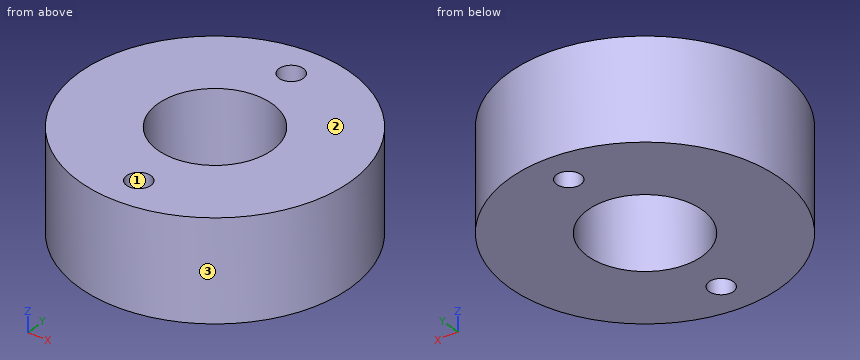
```python
from build123d import *

# Parameters (mm, degrees)
SKETCH1_R                      = 9.45
BOSS_EXTRUDE1_DEPTH            = 7
CUT_EXTRUDE1_REACH             = 17.087
SKETCH2_R                      = 4
TAP_DRILL_FOR_M2_5X0_45_TAP1_D = 1.7


with BuildPart() as part:
    # Sketch1 → Boss-Extrude1 (new body)
    with BuildSketch(Plane.XY):
        Circle(SKETCH1_R)
    extrude(amount=BOSS_EXTRUDE1_DEPTH)

    # Sketch2 → Cut-Extrude1 (cut, up to next)
    with BuildSketch(Plane.XY.offset(7), mode=Mode.PRIVATE) as cut_extrude1_sk1:
        Circle(SKETCH2_R)
    cut_extrude1_tool1 = extrude(cut_extrude1_sk1.sketch, amount=-CUT_EXTRUDE1_REACH, mode=Mode.PRIVATE) & part.part
    add(cut_extrude1_tool1.solids().sort_by_distance((0, 0, 7))[0], mode=Mode.SUBTRACT)

    # Tap Drill for M2.5x0.45 Tap1 (through all)
    with Locations(Plane.XY.offset(7)):
        with Locations((0, 7), (0, -7)):
            Hole(TAP_DRILL_FOR_M2_5X0_45_TAP1_D / 2)


solid = part.part
```
Geometry check sheet. Reference: the model listing, model coordinates, mm. Face numbers are marked on the shaded views. Round coordinates to 2 decimals unless told otherwise and drop trailing zeros. Loops run counter-clockwise (first coordinate to the right, second up) from the corner with the lowest first, then second, coordinate; pieces in that order, holes last. Notation, with made-up numbers: (52, 67.5) -> (79, 67.5) arc R13 cw to (79, 79.5) -> close; hole circle Ø10 at (39.5, 40). An arc over 180 degrees is marked (long way). Use a Markdown table: item, result.
(1) Scan lines: probe 1 along Y at (x, z) = (0, 4.5); probe 2 along X at (y, z) = (-7.25, 5.25); probe 3 along X at (y, z) = (2.75, 1). Record each from-to range of solid material in increasing order.
Calculated:
| item | result |
|---|---|
| probe 1 | -9.45 to -7.85, -6.15 to -4, 4 to 6.15, 7.85 to 9.45 |
| probe 2 | -6.06 to -0.81, 0.81 to 6.06 |
| probe 3 | -9.04 to -2.9, 2.9 to 9.04 |
(2) Sectioned sample at C-C (x = -2). Enter the section's corners in (y, z), then the cut area to 3 significant figures.
Calculated:
| item | result |
|---|---|
| outline | (-9.24, 0) -> (-3.46, 0) -> (-3.46, 7) -> (-9.24, 7) -> close; (3.46, 0) -> (9.24, 0) -> (9.24, 7) -> (3.46, 7) -> close |
| area | 80.8 mm² |
(3) Mould release check, pull along Y, two halves, no side actions. Record for the marked faces 1, 2 and 3: released by +Y, released by -Y, zero draft, split by the parting line, or undercut.
Calculated:
| item | result |
|---|---|
| face 1 | undercut |
| face 2 | zero draft |
| face 3 | split by the parting line |
(4) Sectioned sample at B-B (x = 0). Enter the section's corners in (y, z).
Calculated:
| item | result |
|---|---|
| outline | (-9.45, 0) -> (-7.85, 0) -> (-7.85, 7) -> (-9.45, 7) -> close; (-6.15, 0) -> (-4, 0) -> (-4, 7) -> (-6.15, 7) -> close; (4, 0) -> (6.15, 0) -> (6.15, 7) -> (4, 7) -> close; (7.85, 0) -> (9.45, 0) -> (9.45, 7) -> (7.85, 7) -> close |
(5) Sectioned sample at D-D (z = 2). Enter the section's corners in (x, y).
Calculated:
| item | result |
|---|---|
| outline | circle Ø18.9 at (0, 0); hole circle Ø8 at (0, 0); hole circle Ø1.7 at (0, -7); hole circle Ø1.7 at (0, 7) |
(6) Go/stop test with flat-tipped pins: P1, Ø1, axis at y = -1, z = 4.5, coming from the -X side; P2, Ø4, axis at y = 7.5, z = 6, coming from the +X side; P3, Ø1, axis at y = -4, z = 3, coming from the -X side. Record where each tip stops, or that it passes through.
Calculated:
| item | result |
|---|---|
| P1 | x = -9.44 |
| P2 | x = 7.68 |
| P3 | x = -8.78 |
(7) Sectioned sample at A-A (y = 0). Enter the section's corners in (x, z).
Calculated:
| item | result |
|---|---|
| outline | (-9.45, 0) -> (-4, 0) -> (-4, 7) -> (-9.45, 7) -> close; (4, 0) -> (9.45, 0) -> (9.45, 7) -> (4, 7) -> close |
